Source: CAD feature listing. Evaluate the final solid. Frame: model axes, mm. Face numbers are marked on the shaded views. A direction names the side the tool comes from. Give positions to 0.01 mm unless a question says otherwise; leave off trailing zeros. Loops run counter-clockwise (first coordinate to the right, second up) from the corner with the lowest first, then second, coordinate; pieces in that order, holes last. Notation, with made-up numbers: M 60,-18 L 104,-18 A11 cw 104,-11 Z; hole C 13.25,-21.5 d1. An arc over 180 degrees is marked long. Put each result on its own line as item: value. Start each with the question number.
```python
from build123d import *


with BuildPart() as part:
    # Sketch → Revolution (revolve)
    with BuildSketch(Plane.YZ):
        Polygon((0, 0), (0, 650), (-50.522072, 650), (-204.838623, 479.859444), (-205.380112, 411.197937), (-190.189499, 411.197937), (-190.189499, 462.693711), (-19.438213, 626.926208), (-19.438213, 16.230762), (-182.847931, 16.230762), (-181.744675, 0), align=None)
    revolve(axis=Axis((0, 0, 0), (0, 0, 1)))


solid = part.part
```
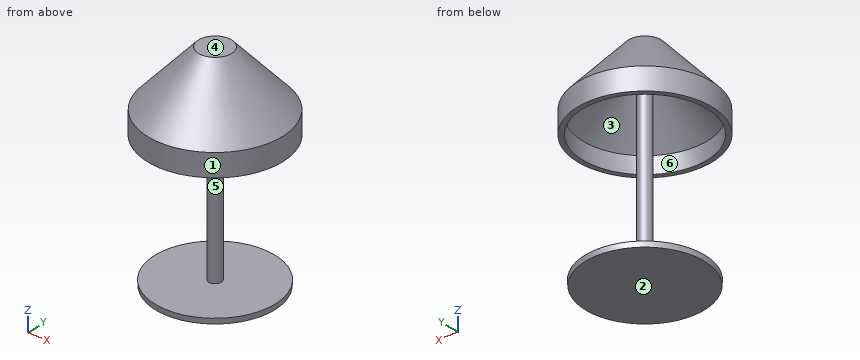
1. Section A-A, the plane z = 498.5. Output: boundary loops of the cut face in (x, y).
2. Pull-direction query (Z, two-part tool) for the marked faces 1, 2 and 3; classes: released by +Z, released by -Z, zero draft, split by the parting line, or undercut.
3. Contact query for flat-ended pins moving along their axis: pin 1 (1.5 mm diameter, centred on y = 16, z = 364.5, fed in from +X); pin 2 (3 mm diameter, centred on x = -108.5, y = -153.5, fed in from -Z); pin 3 (12 mm diameter, centred on x = 100.5, y = 84, fed in from +Z); pin 4 (1.5 mm diameter, centred on x = 74, y = -147, fed in from -Z). Output: stop coordinate, or through.
4. Ray query, line 1 (X direction, y = 0, z = 447.5); line 2 (X direction, y = -11, z = 541); line 3 (Z direction, x = 23, y = -32). Return the intervals inside material, ascending.
5. Set-up query: the marked faces 4, 5 and 6. Return all of +Z, -Z, +X, -X, +Y, -Y with unobstructed straight access to the full face (end or side cutting, diameter ignored); none if empty.
6. Section B-B, the plane z = 192. Output: boundary loops of the cut face in (x, y), plus the area to 3 significant figures.
Results found:
1. outline: C 0,0 d375.86; C 0,0 d38.88; hole C 0,0 d305.92
2. face 1: released by +Z
2. face 2: released by -Z
2. face 3: undercut
3. pin 1: x = 12.05
3. pin 2: z = 463.38
3. pin 3: z = 567.9
3. pin 4: z = 0
4. line 1: -205.09 to -190.19, -19.44 to 19.44, 190.19 to 205.09
4. line 2: -148.98 to -108.22, -16.03 to 16.03, 108.22 to 148.98
4. line 3: 0 to 16.23, 607.72 to 650
5. face 4: +Z, +X, -X, +Y, -Y
5. face 5: none
5. face 6: -Z
6. outline: C 0,0 d38.88
6. area: 1,190 mm²
